```python
from build123d import *

# Parameters (mm, degrees)
SKETCH2_W           = 74
SKETCH2_H           = 74
SKETCH2_W_2         = 54
SKETCH2_H_2         = 54
BOSS_EXTRUDE1_DEPTH = 3
SKETCH3_W           = 10
SKETCH3_H           = 25
BOSS_EXTRUDE2_DEPTH = 3
CUT_EXTRUDE1_DEPTH  = 3
BOSS_EXTRUDE3_DEPTH = 3
CUT_EXTRUDE2_DEPTH  = 3
CUT_EXTRUDE3_DEPTH  = 3
CUT_EXTRUDE4_DEPTH  = 3
BOSS_EXTRUDE4_DEPTH = 3
CUT_EXTRUDE6_DEPTH  = 3
SKETCH12_W          = 5
SKETCH12_H          = 28.4
CUT_EXTRUDE7_DEPTH  = 3


with BuildPart() as part:
    # Sketch2 → Boss-Extrude1 (new body)
    with BuildSketch(Plane(origin=(0, 0, 0), x_dir=(0, 0, -1), z_dir=(1, 0, 0))):
        Rectangle(SKETCH2_W, SKETCH2_H)
        Rectangle(SKETCH2_W_2, SKETCH2_H_2, mode=Mode.SUBTRACT)
    extrude(amount=BOSS_EXTRUDE1_DEPTH)

    # Sketch3 → Boss-Extrude2 (add)
    with BuildSketch(Plane(origin=(3, 0, 0), x_dir=(0, 0, -1), z_dir=(1, 0, 0))):
        with Locations((0, 49.5)):
            Rectangle(SKETCH3_W, SKETCH3_H)
    extrude(amount=-BOSS_EXTRUDE2_DEPTH)

    # Sketch4 → Cut-Extrude1 (cut)
    with BuildSketch(Plane.ZY):
        with BuildLine():
            ThreePointArc((-5, 57), (-3.535533906, 60.535533906), (0, 62))
            Line((0, 62), (-5, 62))
            Line((-5, 62), (-5, 57))
        make_face()
        with BuildLine():
            ThreePointArc((0, 62), (3.535533906, 60.535533906), (5, 57))
            Line((5, 57), (5, 62))
            Line((5, 62), (0, 62))
        make_face()
    extrude(amount=-CUT_EXTRUDE1_DEPTH, mode=Mode.SUBTRACT)

    # Sketch6 → Boss-Extrude3 (add)
    with BuildSketch(Plane(origin=(3, 0, 0), x_dir=(0, 0, -1), z_dir=(1, 0, 0))):
        with BuildLine():
            Line((0.000702858, 63.122185539), (-37, 37))
            Line((-37, 37), (-27, 37))
            Line((-27, 37), (-5, 52.531815276))
            Line((-5, 52.531815276), (-5, 57))
            ThreePointArc((-5, 57), (0, 62), (5, 57))
            Line((5, 57), (5, 52.531815276))
            Line((5, 52.531815276), (27, 37))
            Line((27, 37), (37, 37))
            Line((37, 37), (0.000702858, 63.122185539))
        make_face()
    extrude(amount=-BOSS_EXTRUDE3_DEPTH)

    # Sketch7 → Cut-Extrude2 (cut)
    with BuildSketch(Plane.ZY):
        with BuildLine():
            Line((2.883065745, 61.086269119), (-0.000702858, 63.122185539))
            Line((-0.000702858, 63.122185539), (-2.884435016, 61.086217499))
            ThreePointArc((-2.884435016, 61.086217499), (-0.000692829, 62.001640055), (2.883065745, 61.086269119))
        make_face()
    extrude(amount=-CUT_EXTRUDE2_DEPTH, mode=Mode.SUBTRACT)

    # Sketch8 → Cut-Extrude3 (cut)
    with BuildSketch(Plane(origin=(3, 0, 0), x_dir=(0, 0, -1), z_dir=(1, 0, 0))):
        with BuildLine():
            ThreePointArc((-27, -22.542313426), (-32.066565807, -20.638358178), (-37, -18.4120694))
            Line((-37, -18.4120694), (-37, -37))
            Line((-37, -37), (37, -37))
            Line((37, -37), (37, -18.412705326))
            ThreePointArc((37, -18.412705326), (32.066562187, -20.638895004), (27, -22.542753385))
            Line((27, -22.542753385), (27, -27))
            Line((27, -27), (0.00064811, -27))
            Line((0.00064811, -27), (-27, -27))
            Line((-27, -27), (-27, -22.542313426))
        make_face()
    extrude(amount=-CUT_EXTRUDE3_DEPTH, mode=Mode.SUBTRACT)

    # Sketch9 → Cut-Extrude4 (cut)
    with BuildSketch(Plane.ZY):
        Polygon((-2.000648078, 36.539392014), (-5.000648078, 27), (4.994412692, 27), (1.999351922, 36.540943925), (1.999351922, 60.001640055), (-2.000648078, 60.001640055), align=None)
    extrude(amount=-CUT_EXTRUDE4_DEPTH, mode=Mode.SUBTRACT)

    # Sketch10 → Boss-Extrude4 (add)
    with BuildSketch(Plane.ZY):
        with BuildLine():
            Line((-5.000648078, 62.001640055), (-5.000648078, 59.592132084))
            Line((-5.000648078, 59.592132084), (-2.884435016, 61.086217499))
            ThreePointArc((-2.884435016, 61.086217499), (-1.513445616, 61.767292541), (-0.000648078, 62.001640055))
            Line((-0.000648078, 62.001640055), (-5.000648078, 62.001640055))
        make_face()
        with BuildLine():
            ThreePointArc((-2.884435016, 61.086217499), (-4.440182664, 59.301755847), (-5.000648078, 57.001640055))
            ThreePointArc((-5.000648078, 57.001640055), (-4.18394821, 54.263027268), (-2.000648078, 52.41906436))
            Line((-2.000648078, 52.41906436), (-2.000648078, 60.001640055))
            Line((-2.000648078, 60.001640055), (1.999351922, 60.001640055))
            Line((1.999351922, 60.001640055), (1.999351922, 52.41906436))
            ThreePointArc((1.999351922, 52.41906436), (4.182652055, 54.263027268), (4.999351922, 57.001640055))
            ThreePointArc((4.999351922, 57.001640055), (4.438865922, 59.301795581), (2.883065745, 61.086269119))
            ThreePointArc((2.883065745, 61.086269119), (1.512106806, 61.76730608), (-0.000648078, 62.001640055))
            ThreePointArc((-0.000648078, 62.001640055), (-1.513445616, 61.767292541), (-2.884435016, 61.086217499))
        make_face()
        with BuildLine():
            Line((4.999351922, 62.001640055), (-0.000648078, 62.001640055))
            ThreePointArc((-0.000648078, 62.001640055), (1.512106806, 61.76730608), (2.883065745, 61.086269119))
            Line((2.883065745, 61.086269119), (4.999351922, 59.592188848))
            Line((4.999351922, 59.592188848), (4.999351922, 62.001640055))
        make_face()
    extrude(amount=-BOSS_EXTRUDE4_DEPTH)

    # Sketch11 → Cut-Extrude6 (cut)
    with BuildSketch(Plane(origin=(3, 0, 0), x_dir=(0, 0, -1), z_dir=(1, 0, 0))):
        Polygon((-27, -3), (-37, -13), (-37, -22.542313426), (-27, -22.542313426), align=None)
        Polygon((27, -3), (27, -22.542753385), (37, -22.542753385), (37, -13), align=None)
    extrude(amount=-CUT_EXTRUDE6_DEPTH, mode=Mode.SUBTRACT)

    # Sketch12 → Cut-Extrude7 (cut)
    with BuildSketch(Plane(origin=(3, 0, 0), x_dir=(0, 0, -1), z_dir=(1, 0, 0))):
        with Locations((34.5, 12.8)):
            Rectangle(SKETCH12_W, SKETCH12_H)
    extrude(amount=-CUT_EXTRUDE7_DEPTH, mode=Mode.SUBTRACT)


solid = part.part
```
Work out the finished part from the listing and answer in its coordinate system (mm). A direction names the side the tool comes from. Give positions to 0.01 mm unless a question says otherwise; leave off trailing zeros. Loops run counter-clockwise (first coordinate to the right, second up) from the corner with the lowest first, then second, coordinate; pieces in that order, holes last. Notation, with made-up numbers: (70.25, 31.25) -> (98.25, 31.25) arc R20 cw to (98.25, 54.25) -> close; hole circle Ø11 at (64, -29.5). An arc over 180 degrees is marked (long way). One line per question, with ' | ' between items. Start each with the question number.
1) Section A-A, the plane y = 16 is taken. Determine the outline of the cut face in (x, z), then the cut area to 3 significant figures.
2) Section C-C, the plane y = 44 is taken. Determine the outline of the cut face in (x, z).
3) Section B-B, the plane x = 2.4 is taken. Determine the outline of the cut face in (y, z).
4) Each of these flat-tipped pins is pushed along its axis until it touches: pin 1 (1.2 mm diameter, centred on x = 1.5, y = 60.5, fed in from -Z); pin 2 (0.9 mm diameter, centred on x = 1.5, z = -18, fed in from -Y); pin 3 (1.5 mm diameter, centred on x = 2, z = 0, fed in from -Y); pin 4 (5 mm diameter, centred on y = 48.5, z = -24.5, fed in from +X). Where does it stop, or does it pass through?
5) Section D-D, the plane z = 14.5 is taken. Determine the outline of the cut face in (x, y).
6) Straight lines are drawn through the part: L1, parallel to Z at x = 0.95, y = 43.5; L2, parallel to Z at x = 1.55, y = 16; L3, parallel to Z at x = 1.3, y = 41. For each, find the intervals that lie inside material, in ascending order.
7) Determine the mould class of faces 1 (the face through (1.48, 31.7, 3.52)), 2 (the face through (1.52, 48.45, 20.78)), 3 (the face through (2, -1.4, -34)) for opening direction Z: +Z half, -Z half, draft (parallel to the pull), parting line (faces both ways), or undercut.
8) For faces 4 (the face through (1.52, 44.87, -15.85)), 5 (the face through (1, 48, 1.999)), 6 (the face through (1, -7, -37)), 7 (the face through (1, 61, -5.001)), determine the directions among +Z, -Z, +X, -X, +Y, -Y from which every point of the face is accessible in a straight line to the end or side of a thin tool.
Resolved:
1) outline: (0, -32) -> (3, -32) -> (3, -27) -> (0, -27) -> close; (0, 27) -> (3, 27) -> (3, 37) -> (0, 37) -> close | area: 45.0 mm2
2) outline: (0, -27.09) -> (3, -27.09) -> (3, -17.08) -> (0, -17.08) -> close; (0, -5) -> (3, -5) -> (3, -2) -> (0, -2) -> close; (0, 2) -> (3, 2) -> (3, 5) -> (0, 5) -> close; (0, 17.08) -> (3, 17.08) -> (3, 27.08) -> (0, 27.08) -> close
3) outline: (-13, -37) -> (-1.4, -37) -> (-1.4, -32) -> (27, -32) -> (27, -37) -> (37, -37) -> (59.59, -5) -> (62, -5) -> (62, 5) -> (59.59, 5) -> (37, 37) -> (-13, 37) -> (-3, 27) -> (27, 27) -> (27, 4.99) -> (36.54, 2) -> (60, 2) -> (60, -2) -> (36.54, -2) -> (27, -5) -> (27, -27) -> (-3, -27) -> close; hole (37, -27) -> (52.53, -5) -> (37, -5) -> close; hole (37, 5) -> (52.53, 5) -> (37, 27) -> close
4) pin 1: z = -5 | pin 2: y = 27 | pin 3: y = 60 | pin 4: x = 3
5) outline: (0, 27) -> (3, 27) -> (3, 37) -> (0, 37) -> close; (0, 45.82) -> (3, 45.82) -> (3, 52.88) -> (0, 52.88) -> close
6) L1: -27.79 to -17.79, -5 to -2, 2 to 5, 17.79 to 27.79 | L2: -32 to -27, 27 to 37 | L3: -31.33 to -21.33, -5 to -2, 2 to 5, 21.33 to 31.33
7) face 1: undercut | face 2: +Z half | face 3: draft
8) face 4: +X, -X | face 5: +X, -X, -Y | face 6: -Z, +X, -X, +Y, -Y | face 7: -Z, +X, -X, +Y
